Verification items for the finished model (mm, model axes). A direction names the side the tool comes from. Coordinates: 2 decimals unless noted, no trailing zeros. Order: outer loops, then holes, each group sorted by start corner. A loop starts at its lowest first (then second) coordinate and runs counter-clockwise, first axis right, second up. Notation, with made-up numbers: M -13.75,88.25 L 8.25,88.25 A30 ccw 8.25,127.25 Z; hole C 68.5,7.25 d10. An arc over 180 degrees is marked long. Return JSON: item names as keys, results as strings. Group by question number.
Q1. Access from +Z, -Z, +X, -X, +Y, -Y to the whole of each face (thin tool, end or side, straight path). Record for faces 4 (the face through (0, 50, 0)), 5 (the face through (-0.966, -8.656, -1.26)).
Q2. Go/stop test with flat-tipped pins: pin 1 Ø8 at (x, z) = (3, 7.5) entering from -Y; pin 2 Ø12 at (y, z) = (4.5, 9.5) entering from +X; pin 3 Ø10 at (x, y) = (-5.5, 28.5) entering from +Z; pin 4 Ø3 at (x, y) = (5.5, -4.5) entering from -Z. Record where each tip stops, or that it passes through.
Q3. Section check B-B, the plane x = -3.5. Enter the section's corners in (y, z).
Q4. Thickness scan on probe 1 along Y at (x, z) = (-3, 14.5); probe 2 along X at (y, z) = (8, -12.5); probe 3 along X at (y, z) = (21, 5.5). Record the ranges inside material, lowest first.
Q5. Section check A-A, the plane z = 0. Enter the section's corners in (x, y), then the cut area to 3 significant figures.
Q6. Mould release check, pull along Z, two halves, no side actions. Record for faces 1 (the face through (0, 7, 11)), 2 (the face through (-4.88, -0.99, -1.08)), 3 (the face through (0, -2, 2)): pulls with the +Z half, pulls with the -Z half, needs draft (parallel to the pull), parting line crosses it, or undercut.
Q7. Section check D-D, the plane z = 12.5. Enter the section's corners in (x, y), then the cut area to 3 significant figures.
Q8. Section check C-C, the plane y = 24.5. Enter the section's corners in (x, z).
from build123d import *

# Parameters (mm, degrees)
SKETCH1_R           = 17.5
BOSS_EXTRUDE1_DEPTH = 50
SKETCH1_3_R         = 5
BOSS_EXTRUDE2_DEPTH = 2
BOSS_EXTRUDE3_START = -2
SKETCH1_4_R         = 1.5875
BOSS_EXTRUDE3_DEPTH = 13.5
SKETCH1_5_R         = 1.5
CUT_EXTRUDE1_DEPTH  = 13.5


with BuildPart() as part:
    # Sketch1 → Boss-Extrude1 (new body)
    with BuildSketch(Plane(origin=(0, 0, 0), x_dir=(1, 0, 0), z_dir=(0, 1, 0))):
        with Locations(Location((0, 0, 0), (0, 0, 270))):
            Circle(SKETCH1_R)
    extrude(amount=BOSS_EXTRUDE1_DEPTH)

    # Sketch1<3> → Boss-Extrude2 (add)
    with BuildSketch(Plane(origin=(0, 0, 0), x_dir=(1, 0, 0), z_dir=(0, 1, 0))):
        with Locations(Location((0, 0, 0), (0, 0, 270))):
            Circle(SKETCH1_3_R)
    extrude(amount=-BOSS_EXTRUDE2_DEPTH)

    # Sketch1<4> → Boss-Extrude3 (add)
    with BuildSketch(Plane(origin=(0, 0, 0), x_dir=(1, 0, 0), z_dir=(0, 1, 0)).offset(BOSS_EXTRUDE3_START)):
        with Locations(Location((0, 0, 0), (0, 0, 270))):
            Circle(SKETCH1_4_R)
    extrude(amount=-BOSS_EXTRUDE3_DEPTH)

    # Sketch1<5> → Cut-Extrude1 (cut)
    with BuildSketch(Plane(origin=(0, 0, 0), x_dir=(1, 0, 0), z_dir=(0, 1, 0))):
        with Locations(Location((0, -12.5, 0), (0, 0, 270))):
            Circle(SKETCH1_5_R)
        with Locations(Location((0, 12.5, 0), (0, 0, 270))):
            Circle(SKETCH1_5_R)
    extrude(amount=CUT_EXTRUDE1_DEPTH, mode=Mode.SUBTRACT)


solid = part.part
Numbers:
{
 "1": {"face 4": "+Z, -Z, +X, -X, +Y", "face 5": "-Y"},
 "2": {"pin 1": "stops at y = -2", "pin 2": "stops at x = 17.15", "pin 3": "stops at z = 17.49", "pin 4": "passes through"},
 "3": {"outline": "M -2,-3.57 L 0,-3.57 L 0,-17.15 L 50,-17.15 L 50,17.15 L 0,17.15 L 0,3.57 L -2,3.57 Z"},
 "4": {"probe 1": "y = 0 to 50", "probe 2": "x = -12.25 to -1.5, 1.5 to 12.25", "probe 3": "x = -16.61 to 16.61"},
 "5": {"outline": "M -17.5,0 L -5,0 L -5,-2 L -1.59,-2 L -1.59,-15.5 L 1.59,-15.5 L 1.59,-2 L 5,-2 L 5,0 L 17.5,0 L 17.5,50 L -17.5,50 Z", "area": "1,810 mm2"},
 "6": {"face 1": "undercut", "face 2": "parting line crosses it", "face 3": "needs draft"},
 "7": {"outline": "M -12.25,0 L -1.5,0 L -1.5,13.5 L 1.5,13.5 L 1.5,0 L 12.25,0 L 12.25,50 L -12.25,50 Z", "area": "1,180 mm2"},
 "8": {"outline": "C 0,0 d35"}
}
